```python
from build123d import *

# Parameters (mm, degrees)
F1_DEPTH = 5.08
F3_DEPTH = 2.54


with BuildPart() as f1:
    # F0 (on Front) → F1 (new body)
    with BuildSketch(Plane.XZ):
        with BuildLine():
            ThreePointArc((36.0574860958, -3.4041898403), (37.6237458991, 1.2819140519), (37.0658548873, 6.1912416105))
            ThreePointArc((37.0658548873, 6.1912416105), (15.9114920426, 18.7896851438), (0, 0))
            ThreePointArc((0, 0), (-15.9114920426, 18.7896851438), (-37.0658548873, 6.1912416105))
            ThreePointArc((-37.0658548873, 6.1912416105), (-37.6237458991, 1.2819140519), (-36.0574860958, -3.4041898403))
            Line((-36.0574860958, -3.4041898403), (-5.4450800783, -54.4248665362))
            ThreePointArc((-5.4450800783, -54.4248665362), (0, -57.5078184892), (5.4450800783, -54.4248665362))
            Line((5.4450800783, -54.4248665362), (36.0574860958, -3.4041898403))
        make_face()
        Polygon((8.8775694707, -7.6457064603), (8.8775694707, -30.7146664709), (6.1965412883, -30.7146664709), (6.1965412883, -19.8592792915), (-5.9564433354, -19.8592792915), (-5.9564433354, -30.7146664709), (-8.6374715178, -30.7146664709), (-8.6374715178, -7.6457064603), (-5.9564433354, -7.6457064603), (-5.9564433354, -17.4609960774), (6.1965412883, -17.4609960774), (6.1965412883, -7.6457064603), align=None, mode=Mode.SUBTRACT)
    extrude(amount=F1_DEPTH)

    # F2 (on face) → F3 (join)
    with BuildSketch(Plane.XZ.offset(5.08)):
        with BuildLine():
            ThreePointArc((4.0135957961, -42.9156825927), (3.4697843517, -38.8100018767), (-0.2558416024, -40.6188844818))
            ThreePointArc((-0.2558416024, -40.6188844818), (-4.2951963256, -38.8570498508), (-4.5797577389, -43.2547165786))
            Line((-4.5797577389, -43.2547165786), (-0.8440466673, -46.8867695822))
            ThreePointArc((-0.8440466673, -46.8867695822), (0.0773147032, -47.2269785686), (0.9478044693, -46.7721198031))
            Line((0.9478044693, -46.7721198031), (4.0135957961, -42.9156825927))
        make_face()
        with BuildLine():
            ThreePointArc((20.7469986095, 8.5107093396), (18.9506843874, 12.2523134557), (15.2743776915, 10.3258879514))
            ThreePointArc((15.2743776915, 10.3258879514), (10.8884034591, 11.6753417762), (10.1780788442, 7.1417742478))
            Line((10.1780788442, 7.1417742478), (14.230393121, 1.7562222549))
            ThreePointArc((14.230393121, 1.7562222549), (15.9774408389, 1.1327705758), (17.2386550324, 2.4929935292))
            Line((17.2386550324, 2.4929935292), (20.7469986095, 8.5107093396))
        make_face()
        with BuildLine():
            ThreePointArc((-15.0549625712, 7.4408553073), (-15.8788156154, 10.6122074591), (-18.8651549438, 9.2638804494))
            ThreePointArc((-18.8651549438, 9.2638804494), (-22.0074043435, 10.0708263721), (-22.0279623721, 6.8266823587))
            Line((-22.0279623721, 6.8266823587), (-19.3354653916, 2.851523468))
            ThreePointArc((-19.3354653916, 2.851523468), (-18.2623978414, 2.3275004132), (-17.2688172647, 2.9899743876))
            Line((-17.2688172647, 2.9899743876), (-15.0549625712, 7.4408553073))
        make_face()
    extrude(amount=F3_DEPTH)


solid = f1.part
```
Build history of the part. All positions in model axes, mm. A direction names the side the tool comes from. Round coordinates to 2 decimals unless told otherwise and drop trailing zeros. Loops run counter-clockwise (first coordinate to the right, second up) from the corner with the lowest first, then second, coordinate; pieces in that order, holes last.
Item 1: Pin check, flat tips, straight feed: P1, Ø2, axis at x = -13, z = -43, coming from the -Y side; P2, Ø0.8, axis at x = -6.5, y = -2.5, coming from the -Z side; P3, Ø2, axis at x = -6.5, y = -1.5, coming from the +Z side. Stop position of each tip, or through.
Item 2: Saw through at D-D (z = -12). List the corners of the cut face in (x, y).
Item 3: Saw through at A-A (z = -26). List the corners of the cut face in (x, y), then the cut area to 3 significant figures.
Item 4: Two-plate mould, pull along Z, no slides. Class faces 1 (the face through (2.46, -6.33, -44.87)), 2 (the face through (-37.63, -2.5, 1.35)), 3 (the face through (6.197, -3, -25)), 4 (the face through (-19, -7.62, 8)): released by +Z, released by -Z, zero draft, split by the parting line, or undercut.
Item 5: Saw through at C-C (x = -7). List the corners of the cut face in (y, z).
Item 6: Drill centre lines: line 1 along X through (y, z) = (-4.5, -12.5); line 2 along X through (y, z) = (-2.5, -13); line 3 along Y through (x, z) = (14, -2). Where is each one in solid material? Low to high.
Item 7: Saw through at B-B (y = -3.5). List the corners of the cut face in (x, z).
Item 8: Which spindle directions (+Z, -Z, +X, -X, +Y, -Y) get a long thin tool onto all of the face, cutting with end or side? Do faces 5 (the face through (18.97, -6.33, 5.46)), 6 (the face through (-16.18, -6.33, 5.18)), 7 (the face through (15, -7.62, 8)), 8 (the face through (-0.092, -2.504, -57.507)), 9 (the face through (8, -3, -30.715)). Say none if no direction does.
Worked answers:
1. P1: stops at y = -5.08
1. P2: stops at z = -53.33
1. P3: stops at z = 15.15
2. outline: (-30.9, -5.08) - (-8.64, -5.08) - (-8.64, 0) - (-30.9, 0) - close; (-5.96, -5.08) - (6.2, -5.08) - (6.2, 0) - (-5.96, 0) - close; (8.88, -5.08) - (30.9, -5.08) - (30.9, 0) - (8.88, 0) - close
3. outline: (-22.5, -5.08) - (-8.64, -5.08) - (-8.64, 0) - (-22.5, 0) - close; (-5.96, -5.08) - (6.2, -5.08) - (6.2, 0) - (-5.96, 0) - close; (8.88, -5.08) - (22.5, -5.08) - (22.5, 0) - (8.88, 0) - close
3. area: 201 mm2
4. face 1: released by -Z
4. face 2: split by the parting line
4. face 3: undercut
4. face 4: zero draft
5. outline: (-5.08, -51.83) - (0, -51.83) - (0, -30.71) - (-5.08, -30.71) - close; (-5.08, -7.65) - (0, -7.65) - (0, 14.75) - (-5.08, 14.75) - close
6. line 1: x = -30.6 to -8.64, -5.96 to 6.2, 8.88 to 30.6
6. line 2: x = -30.3 to -8.64, -5.96 to 6.2, 8.88 to 30.3
6. line 3: y = -5.08 to 0
7. outline: (-37.07, 6.19) arc R11.43 ccw to (-36.06, -3.4) - (-5.45, -54.42) arc R6.35 ccw to (5.45, -54.42) - (36.06, -3.4) arc R11.43 ccw to (37.07, 6.19) arc R19.05 ccw to (0, 0) arc R19.05 ccw to start; hole (-8.64, -30.71) - (-5.96, -30.71) - (-5.96, -19.86) - (6.2, -19.86) - (6.2, -30.71) - (8.88, -30.71) - (8.88, -7.65) - (6.2, -7.65) - (6.2, -17.46) - (-5.96, -17.46) - (-5.96, -7.65) - (-8.64, -7.65) - close
8. face 5: -Z, +X, -Y
8. face 6: -Z, -Y
8. face 7: +Z, -Z, +X, -X, -Y
8. face 8: -Z, +Y, -Y
8. face 9: +Y, -Y
